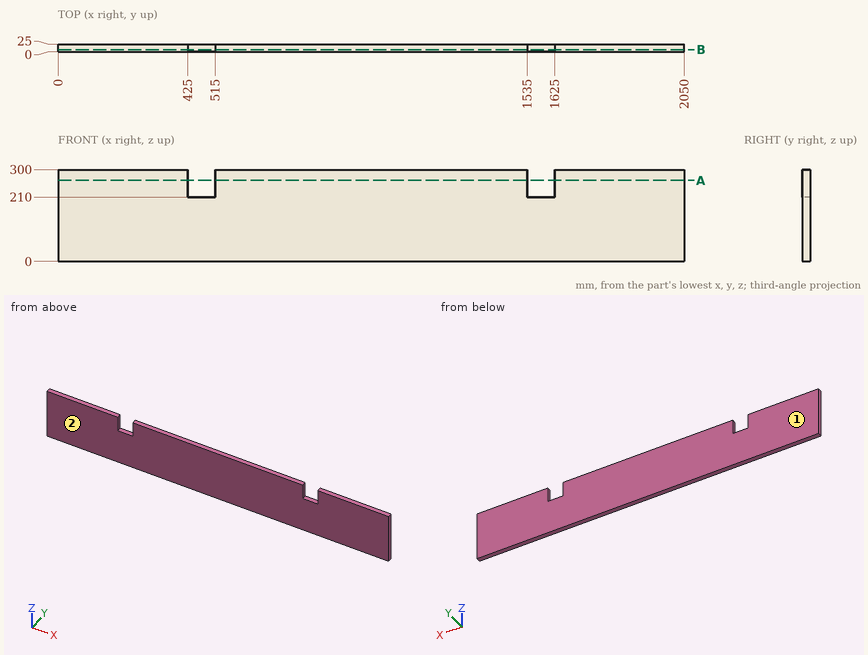
Study the drawing (mm; zero at the part's minimum x, y, z) and answer. Give positions to 0.01 mm unless a question says otherwise; leave off trailing zeros. Write each loop counter-clockwise with the first axis right and the second up, starting at its lowest first coordinate (ties: lowest second). Pieces come first, ordered by that corner, then holes. Notation, with made-up numbers: (16.5, 7) - (58.5, 7) arc R24 ccw to (58.5, 31) - close; hole circle Ø10 at (17, -27.5). An arc over 180 degrees is marked (long way). Write item = value, one per line. Start each with the question number.
Item 1: The mould has two halves that part along Y. Classify the marked faces 1 and 2: +Y half, -Y half, draft (parallel to the pull), parting line (faces both ways), or undercut.
Item 2: Find section A-A (z = 265). Give the vertices of the cut face in (x, y).
Item 3: This flat-tipped pin is pushed along its axis until it touches: P1, Ø12.5, axis at x = 1578.5, y = 15.5, coming from the +Z side. Where does it stop, or does it pass through?
Item 4: Find the intervals of material crossed by probe 1 along X at (y, z) = (20.5, 236); probe 2 along Z at (x, y) = (1577, 12), in increasing order. Write a range as [from, to].
Item 5: Find section B-B (y = 6.5). Give the vertices of the cut face in (x, z).
Response:
q1.face_1 = +Y half
q1.face_2 = -Y half
q2.outline = (0, 0) - (425, 0) - (425, 25) - (0, 25) - close; (515, 0) - (1535, 0) - (1535, 25) - (515, 25) - close; (1625, 0) - (2050, 0) - (2050, 25) - (1625, 25) - close
q3.P1 = 210
q4.probe_1 = [0, 425], [515, 1535], [1625, 2050]
q4.probe_2 = [0, 210]
q5.outline = (0, 0) - (2050, 0) - (2050, 300) - (1625, 300) - (1625, 210) - (1535, 210) - (1535, 300) - (515, 300) - (515, 210) - (425, 210) - (425, 300) - (0, 300) - close
